Answer from the drawing. Dimensions are ordinates in mm from the lowest x, y and z of the part. Give positions to 0.01 mm unless a question says otherwise; leave off trailing zeros. Write each loop counter-clockwise with the first axis right and the second up, starting at its lowest first coordinate (ties: lowest second). Pieces come first, ordered by that corner, then holes. Notation, with made-up numbers: (38, -5.75) -> (66, -5.75) arc R19 ccw to (66, 16.25) -> close; hole circle Ø9 at (49, 47). An arc over 180 degrees is marked (long way). Use a Markdown table: item, result. Add a question column.
Q1. Consider line 1 (Z direction, x = 25.75, y = 9); line 2 (X direction, y = 8, z = 11). Determine where each line is inside the solid, lowest interval first.
Q2. Section B-B, the plane z = 13.5 is taken. Give the vertices of the cut face in (x, y), plus the area to 3 significant figures.
Q3. Section A-A, the plane y = 8.25 is taken. Give the vertices of the cut face in (x, z).
Q4. Each of these flat-tipped pins is pushed along its axis until it touches: pin 1 Ø1.5 at (y, z) = (9, 16.5) entering from +X; pin 2 Ø3.5 at (x, z) = (27, 13.5) entering from +Y. Where does it stop, or does it pass through?
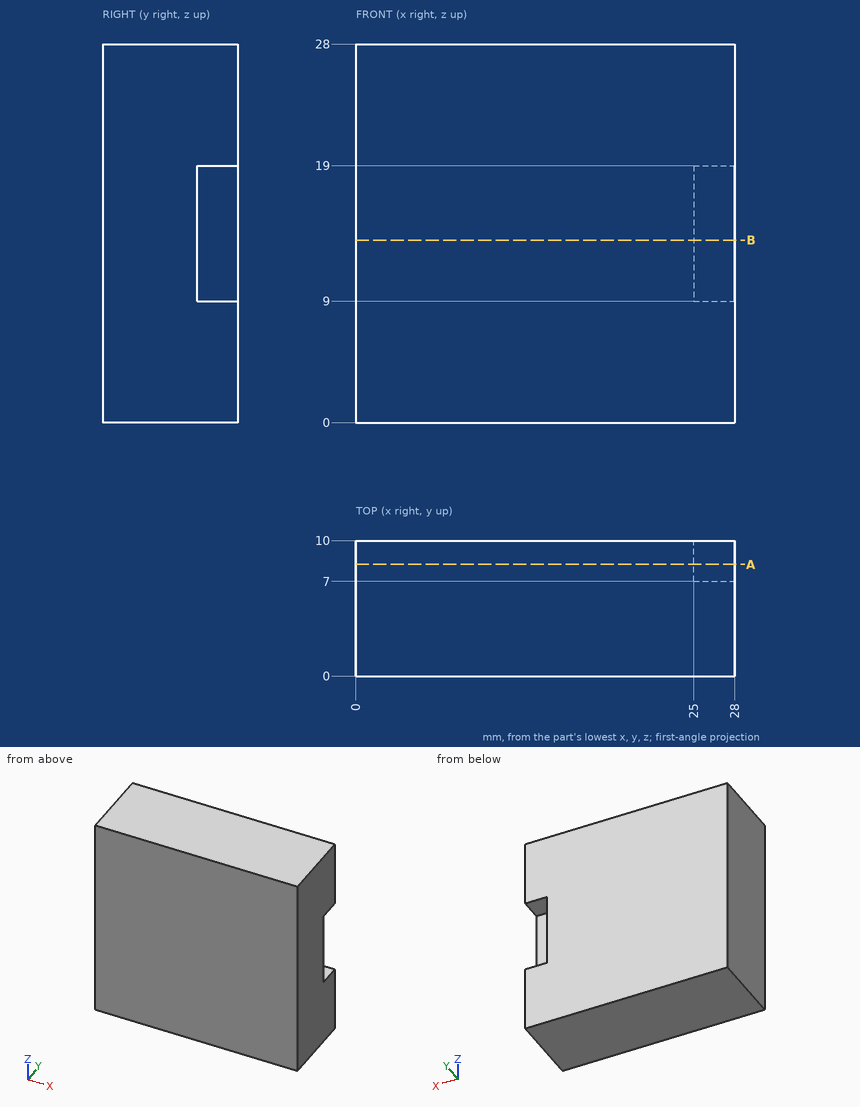
Result set:
| question | item | result |
|---|---|---|
| 1 | line 1 | z = 0 to 9, 19 to 28 |
| 1 | line 2 | x = 0 to 25 |
| 2 | outline | (0, 0) -> (28, 0) -> (28, 7) -> (25, 7) -> (25, 10) -> (0, 10) -> close |
| 2 | area | 271 mm2 |
| 3 | outline | (0, 0) -> (28, 0) -> (28, 9) -> (25, 9) -> (25, 19) -> (28, 19) -> (28, 28) -> (0, 28) -> close |
| 4 | pin 1 | stops at x = 25 |
| 4 | pin 2 | stops at y = 7 |
